Input: part model. Units: mm. Frame: model coordinates. Coordinates: 2 decimals unless noted, no trailing zeros. Write each loop counter-clockwise with the first axis right and the second up, starting at its lowest first coordinate (ties: lowest second). Pieces come first, ordered by that corner, then holes. Notation, with made-up numbers: (45.5, -23.5) -> (79.5, -23.5) arc R11 ccw to (79.5, -8.5) -> close; hole circle Ø10 at (-29.75, -39.75). An arc over 180 degrees is marked (long way). Use one line per item in the form item = value. Start each with the question number.
(1) First-contact query: pin 1 (1.2 mm diameter, centred on x = 137.15, y = -14, fed in from -Z); pin 2 (1.5 mm diameter, centred on y = 27.5, z = 1, fed in from -X); pin 3 (0.9 mm diameter, centred on y = 9.5, z = 2, fed in from +X); pin 4 (1.5 mm diameter, centred on x = 116, z = 1, fed in from -Y). Flat tips, straight axial feed; report the tip coordinate or a pass-through.
(2) Cut plane A-A on y = -23. Return the cut outline in (x, z).
(3) Cut plane C-C on y = 7. Return the cut outline in (x, z), plus the area to 3 significant figures.
(4) Cut plane B-B on x = 79. Return the cut outline in (y, z), plus the area to 3 significant figures.
(5) Cut plane D-D on z = 1. State how many separate pieces and enclosed holes the cut face has, plus the area to 3 significant figures.
(6) Ray query, line 1 along X through (y, z) = (-46.5, 0.9); line 2 along Y through (x, z) = (101, 1.4); line 3 along X through (y, z) = (-18.5, 1.45) (3 decimals). Return the intervals inside material, ascending.
```python
from build123d import *

# Parameters (mm, degrees)
SKETCH1_W           = 281.7
SKETCH1_H           = 140
BOSS_EXTRUDE1_DEPTH = 3
SKETCH2_W           = 110.85
SKETCH2_H           = 20
CUT_EXTRUDE1_DEPTH  = 158.314088689
FILLET1_R           = 2
SKETCH3_W           = 3.7
SKETCH3_H           = 28
CUT_EXTRUDE2_DEPTH  = 158.314088689
SKETCH4_W           = 56.4
SKETCH4_H           = 5
BOSS_EXTRUDE2_DEPTH = 3
FILLET2_R           = 2
SKETCH5_R           = 2
CUT_EXTRUDE3_DEPTH  = 160.601762208
SKETCH6_R           = 1
CUT_EXTRUDE4_DEPTH  = 160.601762208


with BuildPart() as part:
    # Sketch1 → Boss-Extrude1 (new body)
    with BuildSketch(Plane.XY):
        Rectangle(SKETCH1_W, SKETCH1_H)
    extrude(amount=BOSS_EXTRUDE1_DEPTH)

    # Sketch2 → Cut-Extrude1 (cut, through all)
    with BuildSketch(Plane.XY.offset(3)):
        Polygon((-124.75, 45), (-124.75, -20), (-81.525, 12.5), align=None)
        Polygon((-114.75, 55), (-69.875, 21.259398496), (-25, 55), align=None)
        Polygon((-15, 45), (-58.225, 12.5), (-15, -20), align=None)
        Polygon((-69.875, 3.740601504), (-114.75, -30), (-25, -30), align=None)
        with Locations((-70.425, -50)):
            Rectangle(SKETCH2_W, SKETCH2_H)
        with Locations((69.325, -50)):
            Rectangle(SKETCH2_W, SKETCH2_H)
        Polygon((69.875, 3.740601504), (25, -30), (114.75, -30), align=None)
        Polygon((15, 45), (15, -20), (58.225, 12.5), align=None)
        Polygon((25, 55), (69.875, 21.259398496), (114.75, 55), align=None)
        Polygon((124.75, 45), (81.525, 12.5), (124.75, -20), align=None)
    extrude(amount=-CUT_EXTRUDE1_DEPTH, mode=Mode.SUBTRACT)

    # Fillet1
    fillet1_edges = [part.edges().sort_by_distance(p)[0] for p in [
        (114.75, 55, 1.5),
        (25, 55, 1.5),
        (124.75, 45, 1.5),
        (124.75, -20, 1.5),
        (81.525, 12.5, 1.5),
        (-81.525, 12.5, 1.5),
        (-124.75, -20, 1.5),
        (-124.75, 45, 1.5),
        (-25, 55, 1.5),
        (-69.875, 21.259398496, 1.5),
        (-114.75, 55, 1.5),
        (-15, 45, 1.5),
        (-15, -20, 1.5),
        (-58.225, 12.5, 1.5),
        (-69.875, 3.740601504, 1.5),
        (-25, -30, 1.5),
        (-114.75, -30, 1.5),
        (-15, -60, 1.5),
        (-125.85, -60, 1.5),
        (-125.85, -40, 1.5),
        (-15, -40, 1.5),
        (124.75, -60, 1.5),
        (13.9, -60, 1.5),
        (13.9, -40, 1.5),
        (124.75, -40, 1.5),
        (69.875, 3.740601504, 1.5),
        (114.75, -30, 1.5),
        (25, -30, 1.5),
        (15, -20, 1.5),
        (15, 45, 1.5),
    ]]
    fillet(fillet1_edges, radius=FILLET1_R)

    # Sketch3 → Cut-Extrude2 (cut, through all)
    with BuildSketch(Plane.XY.offset(3)):
        with Locations((139, 56)):
            Rectangle(SKETCH3_W, SKETCH3_H)
        with Locations((139, -56)):
            Rectangle(SKETCH3_W, SKETCH3_H)
        with Locations((139, 0)):
            Rectangle(SKETCH3_W, SKETCH3_H)
        with Locations((-139, -28)):
            Rectangle(SKETCH3_W, SKETCH3_H)
        with Locations((-139, 28)):
            Rectangle(SKETCH3_W, SKETCH3_H)
    extrude(amount=-CUT_EXTRUDE2_DEPTH, mode=Mode.SUBTRACT)

    # Sketch4 → Boss-Extrude2 (add)
    with BuildSketch(Plane.XY.offset(3)):
        with Locations((-69.875, -72.5)):
            Rectangle(SKETCH4_W, SKETCH4_H)
        with Locations((69.875, -72.5)):
            Rectangle(SKETCH4_W, SKETCH4_H)
    extrude(amount=-BOSS_EXTRUDE2_DEPTH)

    # Fillet2
    fillet2_edges = [part.edges().sort_by_distance(p)[0] for p in [
        (69.875, 21.259398496, 1.5),
        (58.225, 12.5, 1.5),
    ]]
    fillet(fillet2_edges, radius=FILLET2_R)

    # Sketch5 → Cut-Extrude3 (cut, through all)
    with BuildSketch(Plane(origin=(0, 0, 0), x_dir=(-1, 0, 0), z_dir=(0, 0, -1))):
        with Locations((-5, 62.5)):
            Circle(SKETCH5_R)
    extrude(amount=-CUT_EXTRUDE3_DEPTH, mode=Mode.SUBTRACT)

    # Sketch6 → Cut-Extrude4 (cut, through all)
    with BuildSketch(Plane.XY.offset(3)):
        with Locations((-137.15, 42)):
            Circle(SKETCH6_R)
        with Locations((-137.15, 14)):
            Circle(SKETCH6_R)
        with Locations((-137.15, -14)):
            Circle(SKETCH6_R)
        with Locations((-137.15, -42)):
            Circle(SKETCH6_R)
        with Locations((-98.075, -70)):
            Circle(SKETCH6_R)
        with Locations((-41.675, -70)):
            Circle(SKETCH6_R)
        with Locations((41.675, -70)):
            Circle(SKETCH6_R)
        with Locations((98.075, -70)):
            Circle(SKETCH6_R)
        with Locations((137.15, -42)):
            Circle(SKETCH6_R)
        with Locations((137.15, -14)):
            Circle(SKETCH6_R)
        with Locations((137.15, 14)):
            Circle(SKETCH6_R)
        with Locations((137.15, 42)):
            Circle(SKETCH6_R)
    extrude(amount=-CUT_EXTRUDE4_DEPTH, mode=Mode.SUBTRACT)


solid = part.part
```
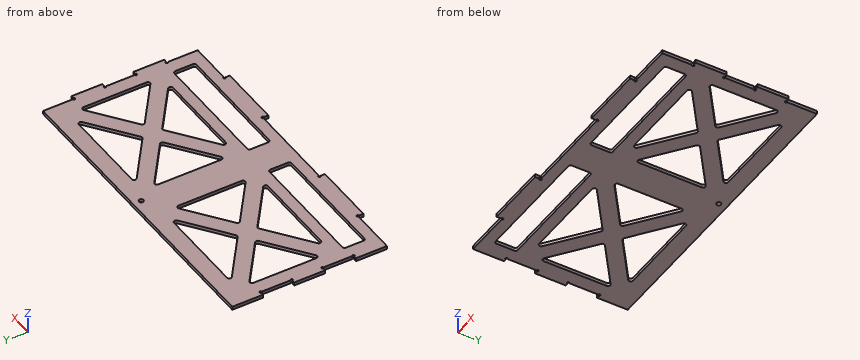
Values:
q1.pin_1 = through
q1.pin_2 = -137.15
q1.pin_3 = 137.15
q1.pin_4 = -70
q2.outline = (-137.15, 0) -> (-105.44, 0) -> (-105.44, 3) -> (-137.15, 3) -> close; (-34.31, 0) -> (34.31, 0) -> (34.31, 3) -> (-34.31, 3) -> close; (105.44, 0) -> (140.85, 0) -> (140.85, 3) -> (105.44, 3) -> close
q3.outline = (-140.85, 0) -> (-124.75, 0) -> (-124.75, 3) -> (-140.85, 3) -> close; (-88.84, 0) -> (-50.91, 0) -> (-50.91, 3) -> (-88.84, 3) -> close; (-15, 0) -> (15, 0) -> (15, 3) -> (-15, 3) -> close; (50.91, 0) -> (88.84, 0) -> (88.84, 3) -> (50.91, 3) -> close; (124.75, 0) -> (137.15, 0) -> (137.15, 3) -> (124.75, 3) -> close
q3.area = 403 mm2
q4.outline = (-75, 0) -> (-60, 0) -> (-60, 3) -> (-75, 3) -> close; (-40, 0) -> (-30, 0) -> (-30, 3) -> (-40, 3) -> close; (-3.12, 0) -> (28.12, 0) -> (28.12, 3) -> (-3.12, 3) -> close; (55, 0) -> (70, 0) -> (70, 3) -> (55, 3) -> close
q4.area = 214 mm2
q5.separate_pieces = 1
q5.enclosed_holes = 11
q5.area = 23,400 mm2
q6.line_1 = -140.85 to -125.85, -15 to 13.9, 124.75 to 137.15
q6.line_2 = -70 to -60, -40 to -30, -19.66 to -2.14, 27.14 to 44.66, 55 to 70
q6.line_3 = -137.15 to -99.455, -40.295 to 40.295, 99.455 to 140.85
